```python
from build123d import *

# Parameters (mm, degrees)
SKETCH_R        = 1.75
SKETCH_W        = 20.5
SKETCH_H        = 51
PAD_DEPTH       = 6
SKETCH001_W     = 23.5
SKETCH001_H     = 54
POCKET_DEPTH    = 3
SKETCH002_W     = 0.8
SKETCH002_H     = 4
PAD001_DEPTH    = 1.4
CHAMFER_SIZE    = 0.59
SKETCH003_W     = 12
SKETCH003_H     = 2
POCKET001_DEPTH = 4.2
SKETCH004_W     = 11
SKETCH004_H     = 2
POCKET002_DEPTH = 1.4
FILLET_R        = 1


with BuildPart() as part:
    # Sketch → Pad (new body)
    with BuildSketch(Plane.XY):
        with BuildLine():
            Line((-13.25, 28.5), (13.25, 28.5))
            Line((13.25, 28.5), (13.25, 3.5))
            Line((15, 3.5), (13.25, 3.5))
            ThreePointArc((15, -3.5), (18.5, 0), (15, 3.5))
            Line((13.25, -3.5), (15, -3.5))
            Line((13.25, -3.5), (13.25, -28.5))
            Line((13.25, -28.5), (-13.25, -28.5))
            Line((-13.25, -28.5), (-13.25, -3.5))
            Line((-15, -3.5), (-13.25, -3.5))
            ThreePointArc((-15, 3.5), (-18.5, 0), (-15, -3.5))
            Line((-13.25, 3.5), (-15, 3.5))
            Line((-13.25, 3.5), (-13.25, 28.5))
        make_face()
        with Locations((-15, 0)):
            Circle(SKETCH_R, mode=Mode.SUBTRACT)
        with Locations((15, 0)):
            Circle(SKETCH_R, mode=Mode.SUBTRACT)
        Rectangle(SKETCH_W, SKETCH_H, mode=Mode.SUBTRACT)
    extrude(amount=PAD_DEPTH)

    # Sketch001 (on Face20 of Pad) → Pocket (cut)
    with BuildSketch(Plane.XY.offset(6)):
        Rectangle(SKETCH001_W, SKETCH001_H)
    extrude(amount=-POCKET_DEPTH, mode=Mode.SUBTRACT)

    # Sketch002 (on Face5 of Pocket) → Pad001 (join)
    with BuildSketch(Plane.XY.offset(6)):
        with Locations((-11.35, 13)):
            Rectangle(SKETCH002_W, SKETCH002_H)
        with Locations((-11.35, -13)):
            Rectangle(SKETCH002_W, SKETCH002_H)
        with Locations((11.35, -13)):
            Rectangle(SKETCH002_W, SKETCH002_H)
        with Locations((11.35, 13)):
            Rectangle(SKETCH002_W, SKETCH002_H)
    extrude(amount=-PAD001_DEPTH)

    # Chamfer
    chamfer_edges = [part.edges().sort_by_distance(p)[0] for p in [
        (-10.95, -13, 4.6),
        (-10.95, -13, 6),
        (-10.95, 13, 4.6),
        (-10.95, 13, 6),
        (10.95, 13, 6),
        (10.95, 13, 4.6),
        (10.95, -13, 6),
        (10.95, -13, 4.6),
    ]]
    chamfer(chamfer_edges, length=CHAMFER_SIZE)

    # Sketch003 (on Face4 of Chamfer) → Pocket001 (cut)
    with BuildSketch(Plane.XY.offset(6)):
        with Locations((0, -28)):
            Rectangle(SKETCH003_W, SKETCH003_H)
    extrude(amount=-POCKET001_DEPTH, mode=Mode.SUBTRACT)

    # Sketch004 (on Face4 of Pocket001) → Pocket002 (cut)
    with BuildSketch(Plane.XY.offset(6)):
        with Locations((0, 28)):
            Rectangle(SKETCH004_W, SKETCH004_H)
    extrude(amount=-POCKET002_DEPTH, mode=Mode.SUBTRACT)

    # Fillet
    fillet_edges = [part.edges().sort_by_distance(p)[0] for p in [
        (-6, -27.75, 1.8),
        (6, -27.75, 1.8),
    ]]
    fillet(fillet_edges, radius=FILLET_R)


solid = part.part
```
Check sheet for the modelled part. Datum: model origin and axes. Units: mm. A direction names the side the tool comes from. Give positions to 0.01 mm unless a question says otherwise; leave off trailing zeros. Order: outer loops, then holes, each group sorted by start corner. A loop starts at its lowest first (then second) coordinate and runs counter-clockwise, first axis right, second up. Notation, with made-up numbers: (-25.5, -7) -> (30.5, -7) arc R31 ccw to (30.5, 30) -> close; hole circle Ø1 at (18.5, -13.75). An arc over 180 degrees is marked (long way). Return JSON: item names as keys, results as strings.
1. Mould release check, pull along Y, two halves, no side actions. Record for faces 6 (the flat face through (-11.75, 0, 5)), 7 (the flat face through (11.75, 0, 5)), 8 (the cylindrical face through (-18.5, 0.1, 3)), 9 (the flat face through (5.5, 28, 5)): +Y half, -Y half, draft (parallel to the pull), parting line (faces both ways), or undercut.
From the geometry:
{"face 6": "undercut", "face 7": "undercut", "face 8": "parting line", "face 9": "draft"}
2. Material ranges on probe 1 along Y at (x, z) = (-15, 2.4); probe 2 along Y at (x, z) = (9, 3.2); probe 3 along X at (y, z) = (-11, 0.35), recorded low to high. Write a range as [from, to].
From the geometry:
{"probe 1": "[-3.5, -1.75], [1.75, 3.5]", "probe 2": "[-28.5, -27], [27, 28.5]", "probe 3": "[-13.25, -10.25], [10.25, 13.25]"}
3. Cross-section at C-C, the plane y = 13. Record the cut outline in (x, z), plus the area to 3 significant figures.
From the geometry:
{"outline": "(-13.25, 0) -> (-10.25, 0) -> (-10.25, 3) -> (-11.75, 3) -> (-11.75, 4.6) -> (-11.54, 4.6) -> (-10.95, 5.19) -> (-10.95, 5.41) -> (-11.54, 6) -> (-13.25, 6) -> close; (10.25, 0) -> (13.25, 0) -> (13.25, 6) -> (11.54, 6) -> (10.95, 5.41) -> (10.95, 5.19) -> (11.54, 4.6) -> (11.75, 4.6) -> (11.75, 3) -> (10.25, 3) -> close", "area": "28.5 mm^2"}
4. Cross-section at A-A, the plane y = 0. Record the cut outline in (x, z), plus the area to 3 significant figures.
From the geometry:
{"outline": "(-18.5, 0) -> (-16.75, 0) -> (-16.75, 6) -> (-18.5, 6) -> close; (-13.25, 0) -> (-10.25, 0) -> (-10.25, 3) -> (-11.75, 3) -> (-11.75, 6) -> (-13.25, 6) -> close; (10.25, 0) -> (13.25, 0) -> (13.25, 6) -> (11.75, 6) -> (11.75, 3) -> (10.25, 3) -> close; (16.75, 0) -> (18.5, 0) -> (18.5, 6) -> (16.75, 6) -> close", "area": "48.0 mm^2"}
5. Go/stop test with flat-tipped pins: P1, Ø1.9, axis at x = 14, z = 4, coming from the -Y side; P2, Ø1.5, axis at y = 3, z = 5, coming from the -X side; P3, Ø3.5, axis at y = -7.5, z = 2, coming from the -X side; P4, Ø1.5, axis at y = -10, z = 1.5, coming from the +X side. Record where each tip stops, or that it passes through.
From the geometry:
{"P1": "y = -28.5", "P2": "x = -17.68", "P3": "x = -13.25", "P4": "x = 13.25"}
6. Cross-section at D-D, the plane z = 0.8. Record the cut outline in (x, y).
From the geometry:
{"outline": "(-15, -3.5) -> (-13.25, -3.5) -> (-13.25, -28.5) -> (13.25, -28.5) -> (13.25, -3.5) -> (15, -3.5) arc R3.5 ccw to (15, 3.5) -> (13.25, 3.5) -> (13.25, 28.5) -> (-13.25, 28.5) -> (-13.25, 3.5) -> (-15, 3.5) arc R3.5 ccw to start; hole circle Ø3.5 at (-15, 0); hole (-10.25, -25.5) -> (10.25, -25.5) -> (10.25, 25.5) -> (-10.25, 25.5) -> close; hole circle Ø3.5 at (15, 0)"}
7. Set-up check for faces 1 (the flat face through (13.25, 16, 3)), 2 (the flat face through (0, 27, 4)), 3 (the flat face through (0, -27, 2)), 4 (the flat face through (-14, 3.5, 3)), 5 (the flat face through (-14, -3.5, 3)): record each of +Z, -Z, +X, -X, +Y, -Y from which the full face is reachable in a straight line by a thin tool's end or side.
From the geometry:
{"face 1": "+Z, -Z, +X, +Y", "face 2": "+Z", "face 3": "+Z, -Y", "face 4": "+Z, -Z, -X, +Y", "face 5": "+Z, -Z, -X, -Y"}
8. Cross-section at B-B, the plane x = -9. Record the cut outline in (y, z).
From the geometry:
{"outline": "(-28.5, 0) -> (-25.5, 0) -> (-25.5, 3) -> (-27, 3) -> (-27, 6) -> (-28.5, 6) -> close; (25.5, 0) -> (28.5, 0) -> (28.5, 6) -> (27, 6) -> (27, 3) -> (25.5, 3) -> close"}
